```python
from build123d import *

# Parameters (mm, degrees)
BOSS_EXTRUDE1_DEPTH = 22.7
SKETCH2_R           = 2.1
CUT_EXTRUDE1_DEPTH  = 22.7
SKETCH4_W           = 4.5
SKETCH4_H           = 4.5
CUT_EXTRUDE2_DEPTH  = 6.1
SKETCH7_R           = 1.5
CUT_EXTRUDE3_DEPTH  = 13
SKETCH9_R           = 2.4
CUT_EXTRUDE4_DEPTH  = 3
FILLET1_R           = 3
CHAMFER2_SIZE       = 1.428148007
CHAMFER2_SIZE_2     = 1


with BuildPart() as part:
    # Sketch1 → Boss-Extrude1 (new body)
    with BuildSketch(Plane(origin=(0, 0, 0), x_dir=(0, 0, -1), z_dir=(1, 0, 0))):
        Polygon((-12.25, -146.25), (12.25, -146.25), (12.25, -140.25), (12.25, -138.77), (2.91, -138.77), (-2.91, -138.77), (-12.25, -138.77), (-12.25, -140.25), align=None)
    extrude(amount=BOSS_EXTRUDE1_DEPTH)

    # Sketch2 → Cut-Extrude1 (cut)
    with BuildSketch(Plane(origin=(0, -138.77, 0), x_dir=(1, 0, 0), z_dir=(0, 1, 0))):
        with Locations(Location((14.85, 2.91, 0), (0, 0, 270))):
            Circle(SKETCH2_R)
        with Locations(Location((7.85, 2.91, 0), (0, 0, 270))):
            Circle(SKETCH2_R)
        with Locations(Location((14.85, -2.91, 0), (0, 0, 270))):
            Circle(SKETCH2_R)
        with Locations(Location((7.85, -2.91, 0), (0, 0, 270))):
            Circle(SKETCH2_R)
    extrude(amount=-CUT_EXTRUDE1_DEPTH, mode=Mode.SUBTRACT)

    # Sketch4 → Cut-Extrude2 (cut)
    with BuildSketch(Plane.XZ.offset(146.25)):
        with Locations((7.85, 2.91)):
            Rectangle(SKETCH4_W, SKETCH4_H)
        with Locations((14.85, 2.91)):
            Rectangle(SKETCH4_W, SKETCH4_H)
        with Locations((14.85, -2.91)):
            Rectangle(SKETCH4_W, SKETCH4_H)
        with Locations((7.85, -2.91)):
            Rectangle(SKETCH4_W, SKETCH4_H)
    extrude(amount=-CUT_EXTRUDE2_DEPTH, mode=Mode.SUBTRACT)

    # Sketch7 → Cut-Extrude3 (cut)
    with BuildSketch(Plane(origin=(0, -138.77, 0), x_dir=(-1, 0, 0), z_dir=(0, -1, 0))):
        with Locations(Location((-3, -7.28, 0), (0, 0, 270))):
            Circle(SKETCH7_R)
        with Locations(Location((-19.7, -7.28, 0), (0, 0, 270))):
            Circle(SKETCH7_R)
        with Locations(Location((-19.7, 7.25, 0), (0, 0, 270))):
            Circle(SKETCH7_R)
        with Locations(Location((-3, 7.25, 0), (0, 0, 270))):
            Circle(SKETCH7_R)
    extrude(amount=CUT_EXTRUDE3_DEPTH, mode=Mode.SUBTRACT)

    # Sketch9 → Cut-Extrude4 (cut)
    with BuildSketch(Plane(origin=(0, -138.77, 0), x_dir=(1, 0, 0), z_dir=(0, 1, 0))):
        with Locations(Location((3, 7.25, 0), (0, 0, 270))):
            Circle(SKETCH9_R)
        with Locations(Location((19.7, 7.25, 0), (0, 0, 270))):
            Circle(SKETCH9_R)
        with Locations(Location((19.7, -7.28, 0), (0, 0, 270))):
            Circle(SKETCH9_R)
        with Locations(Location((3, -7.28, 0), (0, 0, 270))):
            Circle(SKETCH9_R)
    extrude(amount=-CUT_EXTRUDE4_DEPTH, mode=Mode.SUBTRACT)

    # Fillet1
    # the kernel refuses this fillet: 3 mm, written as the material it takes off along each edge
    with BuildSketch(Plane(origin=(-7.5, -138.77, 12.25), x_dir=(0, -1, 0), z_dir=(1, 0, 0))) as fillet1_piece_1:
        with BuildLine():
            CenterArc((FILLET1_R, FILLET1_R), FILLET1_R, 180, 90)
            Line((0, FILLET1_R), (0, 0))
            Line((0, 0), (FILLET1_R, 0))
        make_face()
    extrude(amount=37.7, mode=Mode.SUBTRACT)
    with BuildSketch(Plane(origin=(-7.5, -138.77, -12.25), x_dir=(0, -1, 0), z_dir=(1, 0, 0))) as fillet1_piece_2:
        with BuildLine():
            CenterArc((FILLET1_R, -FILLET1_R), FILLET1_R, 90, 90)
            Line((0, -FILLET1_R), (0, 0))
            Line((0, 0), (FILLET1_R, 0))
        make_face()
    extrude(amount=37.7, mode=Mode.SUBTRACT)

    # Chamfer2
    # the kernel refuses this chamfer: 1.428148007, 1 mm, written as the material it takes off along each edge
    with BuildSketch(Plane(origin=(7.85, -138.77, 2.91), x_dir=(0, 0, 1), z_dir=(-1, 0, 0))) as chamfer2_piece_1:
        Polygon((2.1 + CHAMFER2_SIZE, 0), (2.1, -CHAMFER2_SIZE_2), (2.1, 0), align=None)
    revolve(axis=Axis((7.85, -138.77, 2.91), (0, 1, 0)), mode=Mode.SUBTRACT)
    with BuildSketch(Plane(origin=(7.85, -138.77, -2.91), x_dir=(0, 0, 1), z_dir=(-1, 0, 0))) as chamfer2_piece_2:
        Polygon((2.1 + CHAMFER2_SIZE, 0), (2.1, -CHAMFER2_SIZE_2), (2.1, 0), align=None)
    revolve(axis=Axis((7.85, -138.77, -2.91), (0, 1, 0)), mode=Mode.SUBTRACT)
    with BuildSketch(Plane(origin=(14.85, -138.77, -2.91), x_dir=(0, 0, 1), z_dir=(-1, 0, 0))) as chamfer2_piece_3:
        Polygon((2.1 + CHAMFER2_SIZE, 0), (2.1, -CHAMFER2_SIZE_2), (2.1, 0), align=None)
    revolve(axis=Axis((14.85, -138.77, -2.91), (0, 1, 0)), mode=Mode.SUBTRACT)
    with BuildSketch(Plane(origin=(14.85, -138.77, 2.91), x_dir=(0, 0, 1), z_dir=(-1, 0, 0))) as chamfer2_piece_4:
        Polygon((2.1 + CHAMFER2_SIZE, 0), (2.1, -CHAMFER2_SIZE_2), (2.1, 0), align=None)
    revolve(axis=Axis((14.85, -138.77, 2.91), (0, 1, 0)), mode=Mode.SUBTRACT)


solid = part.part
```
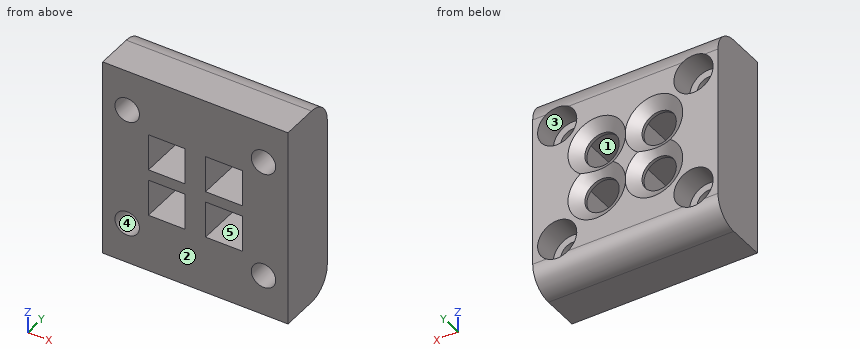
Geometry check sheet. Reference: the model listing, model coordinates, mm. Face numbers are marked on the shaded views. A direction names the side the tool comes from. Coordinates: 2 decimals unless noted, no trailing zeros. Loops run counter-clockwise (first coordinate to the right, second up) from the corner with the lowest first, then second, coordinate; pieces in that order, holes last. Notation, with made-up numbers: (15, 20.5) -> (38, 20.5) arc R25 ccw to (38, 36.5) -> close; hole circle Ø7 at (-26.5, 52). An arc over 180 degrees is marked (long way). Put each result on its own line as item: value.
1) Thickness scan on line 1 (X direction, y = -139.95, z = 2.91); line 2 (X direction, y = -143.5, z = -5); line 3 (Z direction, x = 8, y = -145.5). Record the ranges inside material, lowest first.
Result set:
line 1: x = 0 to 5.75, 9.95 to 12.75, 16.95 to 22.7
line 2: x = 0 to 5.6, 10.1 to 12.6, 17.1 to 22.7
line 3: z = -12.25 to -5.16, -0.66 to 0.66, 5.16 to 12.25
2) Release check for a two-part mould opening along X. For the marked faces 1 and 2 record: released by +X, released by -X, zero draft, split by the parting line, or undercut.
Result set:
face 1: undercut
face 2: zero draft
3) Cross-section at C-C on y = -143. Count the separate pieces of the cut face and the enclosed holes in it, plus the area to 3 significant figures.
Result set:
separate pieces: 1
enclosed holes: 8
area: 447 mm^2
4) Cross-section at B-B on x = 3. Record the boundary of the cut face in (y, z).
Result set:
outline: (-146.25, -12.25) -> (-141.77, -12.25) arc R3 ccw to (-138.8, -9.65) -> (-141.77, -9.65) -> (-141.77, -8.75) -> (-146.25, -8.75) -> close; (-146.25, -5.75) -> (-141.77, -5.75) -> (-141.77, -4.85) -> (-138.77, -4.85) -> (-138.77, 4.88) -> (-141.77, 4.88) -> (-141.77, 5.78) -> (-146.25, 5.78) -> close; (-146.25, 8.78) -> (-141.77, 8.78) -> (-141.77, 9.68) -> (-138.8, 9.68) arc R3 ccw to (-141.77, 12.25) -> (-146.25, 12.25) -> close
5) Cross-section at A-A on z = 7.28. Record the boundary of the cut face in (x, y).
Result set:
outline: (0, -146.25) -> (1.5, -146.25) -> (1.5, -141.77) -> (0.6, -141.77) -> (0.6, -138.77) -> (0, -138.77) -> close; (4.5, -146.25) -> (18.2, -146.25) -> (18.2, -141.77) -> (17.3, -141.77) -> (17.3, -138.77) -> (5.4, -138.77) -> (5.4, -141.77) -> (4.5, -141.77) -> close; (21.2, -146.25) -> (22.7, -146.25) -> (22.7, -138.77) -> (22.1, -138.77) -> (22.1, -141.77) -> (21.2, -141.77) -> close
6) Gauge pin test, flat end, axial feed: pin 1 Ø3.5 at (x, z) = (3, 7.28) entering from +Y. Record the tip position at first contact, or that the pin passes through.
Result set:
pin 1: stops at y = -141.77
7) Tool access check on the marked faces 3, 4 and 5. Record the directions out of +Z, -Z, +X, -X, +Y, -Y that give a thin tool (end or side, any length) a straight path to the whole face; none if there is none.
Result set:
face 3: +Y
face 4: +Y, -Y
face 5: -Y
8) Cross-section at D-D on x = 14.85. Record the boundary of the cut face in (y, z).
Result set:
outline: (-146.25, -12.25) -> (-141.77, -12.25) arc R3 ccw to (-138.77, -9.25) -> (-138.77, -6.44) -> (-139.77, -5.01) -> (-140.15, -5.01) -> (-140.15, -5.16) -> (-146.25, -5.16) -> close; (-146.25, -0.66) -> (-140.15, -0.66) -> (-140.15, -0.81) -> (-139.77, -0.81) -> (-139.2, 0) -> (-139.77, 0.81) -> (-140.15, 0.81) -> (-140.15, 0.66) -> (-146.25, 0.66) -> close; (-146.25, 5.16) -> (-140.15, 5.16) -> (-140.15, 5.01) -> (-139.77, 5.01) -> (-138.77, 6.44) -> (-138.77, 9.25) arc R3 ccw to (-141.77, 12.25) -> (-146.25, 12.25) -> close
